Here's how the part is built. I have some questions about the finished solid (model axes, mm). A direction names the side the tool comes from. Coordinates: 2 decimals unless noted, no trailing zeros. Order: outer loops, then holes, each group sorted by start corner. A loop starts at its lowest first (then second) coordinate and runs counter-clockwise, first axis right, second up. Notation, with made-up numbers: (51, -32.5) -> (74, -32.5) arc R25 ccw to (74, -10.5) -> close; hole circle Ø7 at (-25.5, 79). An arc over 180 degrees is marked (long way). One line per item, written item: value. Start each with the question number.
Autodesk Inventor part; units mm, degrees
ref_plane "Plano inicial" through (0, 0, -25.4) normal (0, 0, 1) x (1, 0, 0)
ref_plane "Plano final" through (0, 0, 2215.4) normal (0, 0, 1) x (1, 0, 0)
ref_plane "Plano de trabajo4" through (25.4, 0, -25.4) normal (-0.7071, 0, -0.7071) x (-0.7071, 0, 0.7071)
ref_plane "Plano inicial" through (0, 0, -25.4) normal (0, 0, 1) x (1, 0, 0)
ref_plane "Plano final" through (0, 0, 2215.4) normal (0, 0, 1) x (1, 0, 0)
sketch "Boceto" plane through (0, 0, 0) normal (0, 0, 1) x (1, 0, 0)
  line L0 (-25.4, -19.05) -> (-25.4, 19.05)
  line L1 (-19.05, 25.4) -> (19.05, 25.4)
  line L2 (25.4, 19.05) -> (25.4, -19.05)
  line L3 (19.05, -25.4) -> (-19.05, -25.4)
  arc A0 (-25.4, -19.05) -> (-19.05, -25.4) centre (-19.05, -19.05) ccw
  arc A1 (-19.05, 25.4) -> (-25.4, 19.05) centre (-19.05, 19.05) ccw
  arc A2 (25.4, 19.05) -> (19.05, 25.4) centre (19.05, 19.05) ccw
  arc A3 (19.05, -25.4) -> (25.4, -19.05) centre (19.05, -19.05) ccw
  arc A4 (-19.05, 22.225) -> (-22.225, 19.05) centre (-19.05, 19.05) ccw
  line L4 (-19.05, 22.225) -> (19.05, 22.225)
  arc A5 (22.225, 19.05) -> (19.05, 22.225) centre (19.05, 19.05) ccw
  line L5 (22.225, 19.05) -> (22.225, -19.05)
  arc A6 (19.05, -22.225) -> (22.225, -19.05) centre (19.05, -19.05) ccw
  line L6 (19.05, -22.225) -> (-19.05, -22.225)
  arc A7 (-22.225, -19.05) -> (-19.05, -22.225) centre (-19.05, -19.05) ccw
  line L7 (-22.225, -19.05) -> (-22.225, 19.05)
  line L8 (0, 37.4012) -> (0, -37.4012) construction
  line L9 (-37.4012, 0) -> (37.4012, 0) construction
  dimension "d10" = 50.8
  dimension "d11" = 50.8
  dimension "d12" = 3.175
  dimension "d15" = 25.4
  dimension "d16" = 25.4
  dimension "d17" = 6.35
extrude "Cuerpo" add sketch "Boceto" along normal up to surface (2240.8 mm away) from surface at -25.4
sketch "Sketch3" plane through (0, 0, 0) normal (0, 0, 1) x (1, 0, 0)
  line L0 (0, 0) -> (10, 0)
ref_plane "Work Plane3" through (0, 0, 0) normal (0, -1, 0) x (1, 0, 0)
ref_plane "Plano de trabajo4" through (25.4, 0, -25.4) normal (-0.7071, 0, -0.7071) x (-0.7071, 0, 0.7071)
split "Dividir1" plane through (25.4, 0, -25.4) removes the side toward (-0.7071, 0, -0.7071)
ref_plane "Plano de trabajo5" through (25.4, 0, 2215.4) normal (-0.7071, 0, 0.7071) x (0.7071, 0, 0.7071)
split "Dividir2" plane through (25.4, 0, 2215.4) removes the side toward (-0.7071, 0, 0.7071)
sketch "Boceto5" plane through (19.05, 25.4, 2209.05) normal (0, 1, 0) x (1, 0, 0)
  line L0 (-19.05, 2209.05) -> (-19.05, 19.05)
  line L1 (-38.1, 38.1) -> (0, 0)
  circle A0 centre (-19.05, 1345.45) radius 9.017
  circle A1 centre (-19.05, 558.05) radius 9.017
  line L2 (0, 2228.1) -> (-38.1, 2190)
  circle A2 centre (-19.05, 2113.9013) radius 8.4404
  point P0 (-19.05, 2209.05)
  point P1 (-19.05, 2209.05)
  point P2 (-19.05, 2209.05)
  dimension "d20" = 18.034
  dimension "d21" = 18.034
  dimension "d22" = 863.6
  dimension "d23" = 1651
  dimension "d26" = 95.1487
extrude "Extrusión2" cut sketch "Boceto5" against normal blind 6.35 contours A1 L0 | L0 A1 | A0 L0 | L0 A0
sketch "Sketch4" plane through (0, 0, 0) normal (0, -1, 0) x (1, 0, 0)
  line L0 (-2, -25.4) -> (12, -25.4)
  line L1 (-2, 2215.4) -> (12, 2215.4)
  dimension "d19" = 2240.8
equation "\"d10\" = G_H"
equation "\"d11\" = G_W"
equation "\"d12\" = G_T"
equation "\"d15\" = 0.5 * d10"
equation "\"d16\" = 0.5 * d11"
equation "\"d17\" = G_IR"
equation "\"d3\" = G_L"
equation "\"G_W\" = 50.8"
equation "\"G_H\" = 50.8"
equation "\"G_T\" = 3.175"
equation "\"G_IR\" = 6.35"
equation "\"G_L\" = d19"
equation "\"G_OFFSET_START\" = 25.4"
equation "\"G_OFFSET_END\" = 25.4"
equation "\"d13\" = -G_OFFSET_START"
equation "\"d14\" = G_OFFSET_END + B_L"
equation "\"B_L\" = 2190"
properties part number "AISC - 2 x 2 x 1/8 - 88,22" material "Acero, suave"
Q1. Imagine slicing it at A-A (y = -8). Write out the boundary of the cut face in (x, z) (3 decimals), plus the area to 3 significant figures.
Q2. If we mould it in two halves opening along X, with no side actions, what happens to faces 1 (the face through (0, -25.4, 1079)), 2 (the face through (0, 22.225, 1079)), 3 (the face through (1.8, 22.5, 2191.8))? For each: +X half, -X half, draft (parallel to the pull), parting line (faces both ways), or undercut.
Q3. For faces 4 (the face through (22.225, 0, 1079)), 5 (the face through (25.4, 0, 1079)), which set-ups out of +Z, -Z, +X, -X, +Y, -Y let a thin tool reach every point of the face, with its end or its side?
Q4. I need wall thicknesses on line 1 (X direction, y = -9, z = 513) (3 decimals); line 2 (Z direction, x = 0, y = 23). Which ranges of each line are inside material? Lowest first, please.
Q5. Imagine slicing it at C-C (z = 1957). Write out the boundary of the cut face in (x, y) (3 decimals).
Q6. Imagine slicing it at B-B (x = 0). Write out the boundary of the cut face in (y, z) (3 decimals), plus the area to 3 significant figures.
Q7. For P1, Ø10, axis at x = 17.5, y = -0.5, coming from the -Z side, with a flat end and sliding along its axis, tell me the tip position at first contact or that it passes through.
Completed:
1. outline: (-25.4, 25.4) -> (-22.225, 22.225) -> (-22.225, 2167.775) -> (-25.4, 2164.6) -> close; (22.225, -22.225) -> (25.4, -25.4) -> (25.4, 2215.4) -> (22.225, 2212.225) -> close
1. area: 13,900 mm2
2. face 1: draft
2. face 2: undercut
2. face 3: -X half
3. face 4: +Z, -Z
3. face 5: +Z, -Z, +X, +Y, -Y
4. line 1: x = -25.4 to -22.225, 22.225 to 25.4
4. line 2: z = 0 to 854.58, 872.62 to 1641.98, 1660.02 to 2190
5. outline: (-25.4, -19.05) arc R6.35 ccw to (-19.05, -25.4) -> (19.05, -25.4) arc R6.35 ccw to (25.4, -19.05) -> (25.4, 19.05) arc R6.35 ccw to (19.05, 25.4) -> (-19.05, 25.4) arc R6.35 ccw to (-25.4, 19.05) -> close; hole (-22.225, -19.05) arc R3.175 ccw to (-19.05, -22.225) -> (19.05, -22.225) arc R3.175 ccw to (22.225, -19.05) -> (22.225, 19.05) arc R3.175 ccw to (19.05, 22.225) -> (-19.05, 22.225) arc R3.175 ccw to (-22.225, 19.05) -> close
6. outline: (-25.4, 0) -> (-22.225, 0) -> (-22.225, 2190) -> (-25.4, 2190) -> close; (22.225, 0) -> (25.4, 0) -> (25.4, 854.583) -> (22.225, 854.583) -> close; (22.225, 872.617) -> (25.4, 872.617) -> (25.4, 1641.983) -> (22.225, 1641.983) -> close; (22.225, 1660.017) -> (25.4, 1660.017) -> (25.4, 2190) -> (22.225, 2190) -> close
6. area: 13,800 mm2
7. P1: stops at z = -22.5
